Answer from the drawing. Dimensions are ordinates in mm from the lowest x, y and z of the part. Give positions to 0.01 mm unless a question says otherwise; leave off trailing zeros. Write each loop counter-clockwise with the first axis right and the second up, starting at its lowest first coordinate (ties: lowest second). Pieces come first, ordered by that corner, then holes. Notation, with made-up numbers: (87, -27.75) -> (118, -27.75) arc R34 cw to (118, 6.25) -> close; hole circle Ø5 at (32.25, 5.25). An arc over 180 degrees is marked (long way). Write item = value, one per line.
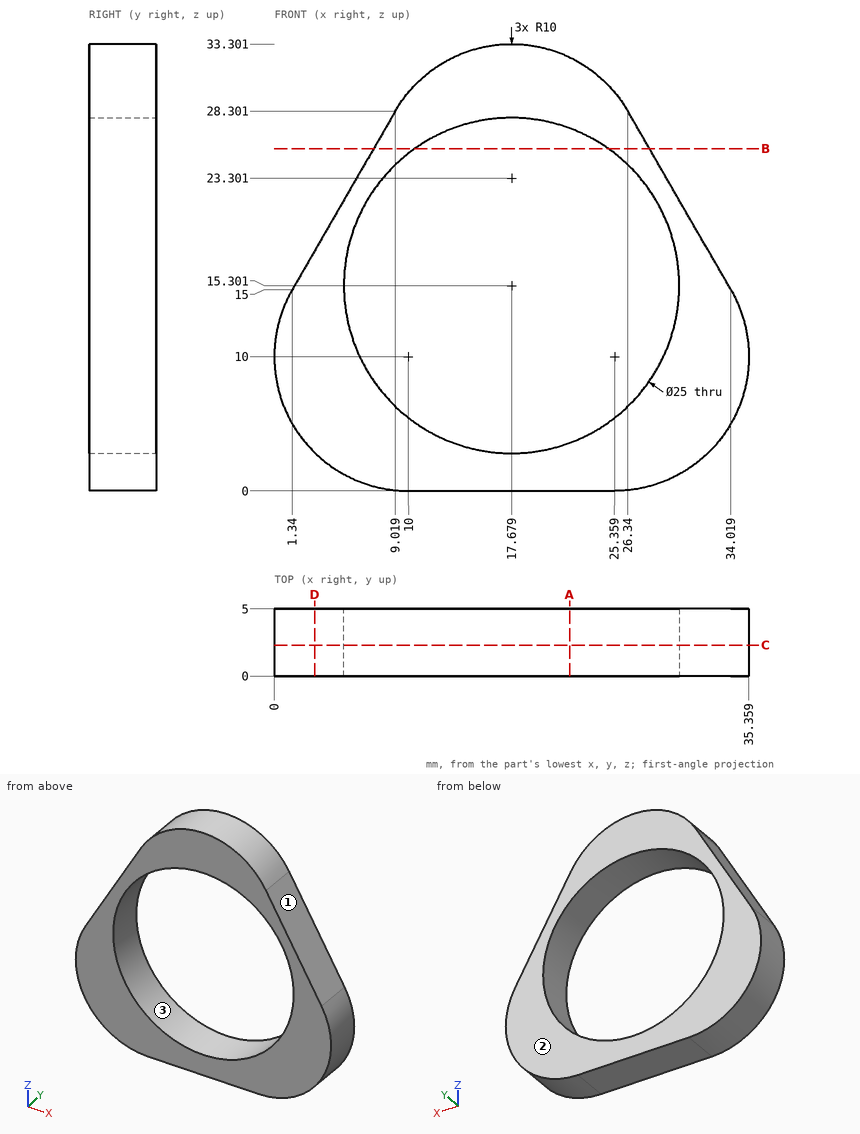
(1) The part is cut by section A-A on x = 22. Determine the outline of the cut face in (y, z).
Checks:
outline = (0, 0) -> (5, 0) -> (5, 3.57) -> (0, 3.57) -> close; (0, 27.03) -> (5, 27.03) -> (5, 32.32) -> (0, 32.32) -> close
(2) The part is cut by section D-D on x = 3. Determine the outline of the cut face in (y, z) (1 decimal).
Checks:
outline = (0, 2.9) -> (5, 2.9) -> (5, 17.9) -> (0, 17.9) -> close
(3) The part is cut by section C-C on y = 2.3. Determine the outline of the cut face in (x, z), plus the area to 3 significant figures.
Checks:
outline = (1.34, 15) arc R10 ccw to (10, 0) -> (25.36, 0) arc R10 ccw to (34.02, 15) -> (26.34, 28.3) arc R10 ccw to (9.02, 28.3) -> close; hole circle Ø25 at (17.68, 15.3)
area = 386 mm²
(4) For a pull along Z with two mould halves and no side action, classify the marked faces 1, 2 and 3 as released by +Z, released by -Z, zero draft, split by the parting line, or undercut.
Checks:
face_1 = released by +Z
face_2 = zero draft
face_3 = undercut
(5) The part is cut by section B-B on z = 25.5. Determine the outline of the cut face in (x, y).
Checks:
outline = (7.4, 0) -> (10.45, 0) -> (10.45, 5) -> (7.4, 5) -> close; (24.91, 0) -> (27.96, 0) -> (27.96, 5) -> (24.91, 5) -> close
(6) Given P1, Ø2, axis at y = 2.5, z = 27.5, coming from the -X side, flat-ended and moving along its own axis, determine where the tip first touches the part or whether it passes through.
Checks:
P1 = 7.98
(7) Consider L1, parallel to Z at x = 17.5, y = 4.5; L2, parallel to Z at x = 8, y = 0.3 (1 decimal); L3, parallel to X at y = 1.4, z = 7.5 (1 decimal). Determine where each line is inside the solid, lowest interval first.
Checks:
L1 = 0 to 2.8, 27.8 to 33.3
L2 = 0.2 to 7.4, 23.2 to 26.5
L3 = 0.3 to 7.9, 27.4 to 35
